Model file for the job. Use its own axes, mm. Face numbers are marked on the shaded views. A direction names the side the tool comes from. Give positions to 0.01 mm unless a question says otherwise; leave off trailing zeros. Loops run counter-clockwise (first coordinate to the right, second up) from the corner with the lowest first, then second, coordinate; pieces in that order, holes last. Notation, with made-up numbers: M 78.5,89.5 L 116.5,89.5 A14 ccw 116.5,115.5 Z; hole C -21.75,-23 d1. An arc over 180 degrees is marked long. Answer in a Markdown table with one row per item.
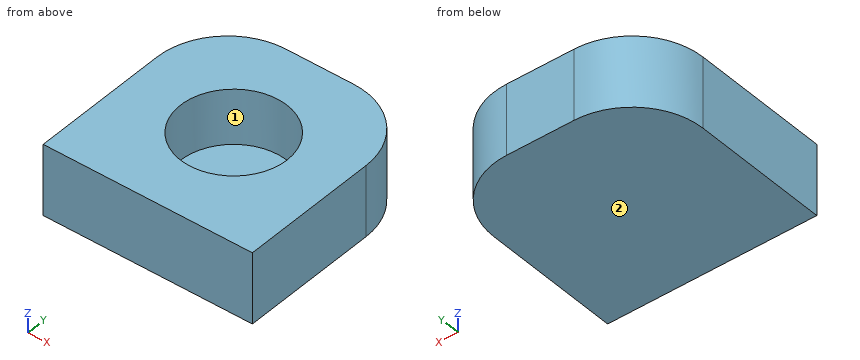
```python
from build123d import *

# Parameters (mm, degrees)
SKETCH1_W           = 11.8
SKETCH1_H           = 11.8
BOSS_EXTRUDE1_DEPTH = 4
SKETCH2_R           = 3
CUT_EXTRUDE1_DEPTH  = 3.1
FILLET1_R           = 4


with BuildPart() as part:
    # Sketch1 → Boss-Extrude1 (new body)
    with BuildSketch(Plane.XY):
        with Locations((5.9, 5.9)):
            Rectangle(SKETCH1_W, SKETCH1_H)
    extrude(amount=BOSS_EXTRUDE1_DEPTH)

    # Sketch2 → Cut-Extrude1 (cut)
    with BuildSketch(Plane.XY.offset(4)):
        with Locations((5.9, 5.9)):
            Circle(SKETCH2_R)
    extrude(amount=-CUT_EXTRUDE1_DEPTH, mode=Mode.SUBTRACT)

    # Fillet1
    fillet1_edges = [part.edges().sort_by_distance(p)[0] for p in [
        (0, 11.8, 2),
        (11.8, 11.8, 2),
    ]]
    fillet(fillet1_edges, radius=FILLET1_R)


solid = part.part
```
Q1. 3-axis set-ups, long thin cutter, end or side, ignore diameter. For the marked faces 1 and 2: which of +Z, -Z, +X, -X, +Y, -Y reach the whole face in a straight line?
Reported:
| item | result |
|---|---|
| face 1 | +Z |
| face 2 | -Z, +X, -X, +Y, -Y |
Q2. Saw through at B-B (y = 5.9). Give the cut face in (x, z).
Reported:
| item | result |
|---|---|
| outline | M 0,0 L 11.8,0 L 11.8,4 L 8.9,4 L 8.9,0.9 L 2.9,0.9 L 2.9,4 L 0,4 Z |
Q3. Saw through at A-A (z = 1.9). Give the cut face in (x, y).
Reported:
| item | result |
|---|---|
| outline | M 0,0 L 11.8,0 L 11.8,7.8 A4 ccw 7.8,11.8 L 4,11.8 A4 ccw 0,7.8 Z; hole C 5.9,5.9 d6 |
Q4. Probe probe 1 along X at (y, z) = (6, 1.7); probe 2 along Z at (x, y) = (7.25, 7.75). List the from-to ranges inside material, lowest first.
Reported:
| item | result |
|---|---|
| probe 1 | 0 to 2.9, 8.9 to 11.8 |
| probe 2 | 0 to 0.9 |
Q5. Drop flat-ended pins along their axis: pin 1 (1.5 mm diameter, centred on y = 9, z = 2, fed in from +X); pin 2 (5 mm diameter, centred on x = 6, y = 6, fed in from +Z); pin 3 (1 mm diameter, centred on y = 10.5, z = 1, fed in from -X). Give the stop position or say it passes through.
Reported:
| item | result |
|---|---|
| pin 1 | x = 11.77 |
| pin 2 | z = 0.9 |
| pin 3 | x = 0.66 |
